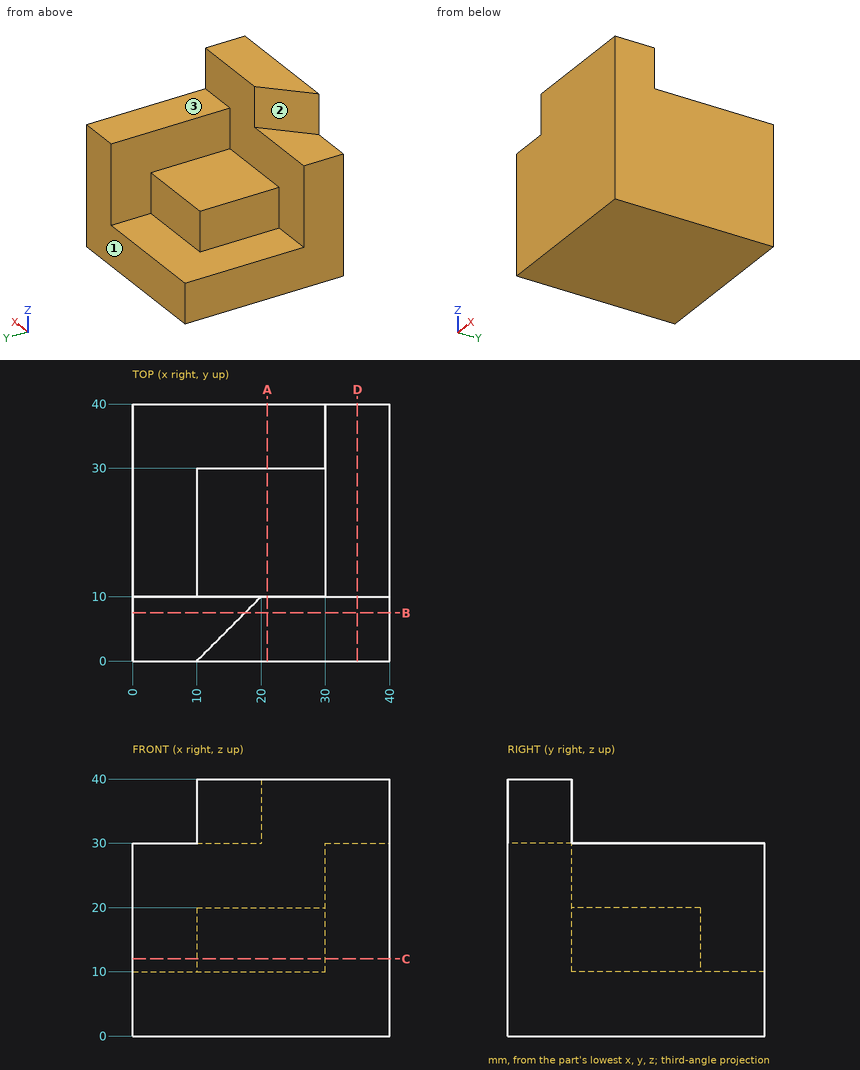
Input: dimensioned drawing with shaded views. Units: mm. Origin: part minimum x, y, z. A direction names the side the tool comes from. Give positions to 0.01 mm unless a question says otherwise; leave off trailing zeros. Write each loop counter-clockwise with the first axis right and the second up, starting at its lowest first coordinate (ties: lowest second). Pieces come first, ordered by that corner, then holes. Notation, with made-up numbers: (34, 30) -> (58, 30) arc R3 ccw to (58, 35) -> close; hole circle Ø9 at (63.25, 27). An arc over 180 degrees is marked (long way). Return JSON: item names as keys, results as strings. Group by question number.
1. Section B-B, the plane y = 7.5. Output: boundary loops of the cut face in (x, z), then the cut area to 4 significant figures.
2. Access query for the marked faces 1, 2 and 3. Directions: +Z, -Z, +X, -X, +Y, -Y. A direction counts if a zero-diameter tool reaches every point of the face in a straight line with its end or side. Return the directions, or none.
3. Section D-D, the plane x = 35. Output: boundary loops of the cut face in (y, z).
4. Section C-C, the plane z = 12. Output: boundary loops of the cut face in (x, y), then the cut area to 3 significant figures.
5. Pin query (flat end, axial travel): pin 1 Ø16 at (x, y) = (24, 25) entering from +Z; pin 2 Ø3 at (y, z) = (19, 17.5) entering from -X; pin 3 Ø9 at (x, z) = (23.5, 31.5) entering from +Y. Return the tip coordinate at first contact, or that it passes through.
6. Material intervals for line 1 (Z direction, x = 17, y = 16); line 2 (Z direction, x = 14, y = 7); line 3 (X direction, y = 20, z = 28), sorted ascending. Write a range as from..to.
7. Section A-A, the plane x = 21. Output: boundary loops of the cut face in (y, z).
Determined:
{
 "1": {"outline": "(0, 0) -> (40, 0) -> (40, 40) -> (17.5, 40) -> (17.5, 30) -> (0, 30) -> close", "area": "1,425 mm2"},
 "2": {"face 1": "+Z, -Z, +X, -X, +Y", "face 2": "+Z, -X, +Y", "face 3": "+Z, +X, -X, +Y"},
 "3": {"outline": "(0, 0) -> (40, 0) -> (40, 30) -> (10, 30) -> (10, 40) -> (0, 40) -> close"},
 "4": {"outline": "(0, 0) -> (40, 0) -> (40, 40) -> (30, 40) -> (30, 30) -> (10, 30) -> (10, 10) -> (0, 10) -> close", "area": "1,100 mm2"},
 "5": {"pin 1": "stops at z = 30", "pin 2": "stops at x = 10", "pin 3": "stops at y = 10"},
 "6": {"line 1": "z = 0..20", "line 2": "z = 0..30", "line 3": "x = 30..40"},
 "7": {"outline": "(0, 0) -> (40, 0) -> (40, 10) -> (30, 10) -> (30, 20) -> (10, 20) -> (10, 40) -> (0, 40) -> close"}
}
